Design review of the part built by this model. Coordinates are the model's own, in mm. A direction names the side the tool comes from. Coordinates: 2 decimals unless noted, no trailing zeros. Order: outer loops, then holes, each group sorted by start corner. A loop starts at its lowest first (then second) coordinate and runs counter-clockwise, first axis right, second up. Notation, with made-up numbers: M 82.25,27.5 L 115.25,27.5 A22 cw 115.25,41.5 Z; hole C 49.5,47 d6. An arc over 180 degrees is marked long. Answer as a JSON object with one key per item and string values.
from build123d import *

# Parameters (mm, degrees)
BOSS_EXTRUDE1_DEPTH = 50
CUT_EXTRUDE1_DEPTH  = 48
FILLET1_R           = 1
FILLET2_R           = 2
SKETCH3_R           = 1.6
CUT_EXTRUDE2_DEPTH  = 1067.768955656


with BuildPart() as part:
    # Sketch1 → Boss-Extrude1 (new body)
    with BuildSketch(Plane(origin=(0, 0, 0), x_dir=(1, 0, 0), z_dir=(0, 1, 0))):
        Polygon((1026.361248777, 29.83084978), (1061.002264928, 49.83084978), (1061.002264928, 99.83084978), (1049.002264928, 99.83084978), (1049.002264928, 56.75905301), (1026.361248777, 43.68725624), align=None)
    extrude(amount=BOSS_EXTRUDE1_DEPTH)

    # Sketch2 → Cut-Extrude1 (cut)
    with BuildSketch(Plane(origin=(0, 50, 0), x_dir=(1, 0, 0), z_dir=(0, 1, 0))):
        Polygon((1059.002264928, 99.83084978), (1059.002264928, 50.985550318), (1026.361248777, 32.140250857), (1013.240003321, 83.162287717), (1049.002264928, 102.282604927), align=None)
    extrude(amount=-CUT_EXTRUDE1_DEPTH, mode=Mode.SUBTRACT)

    # Fillet1
    fillet1_edges = [part.edges().sort_by_distance(p)[0] for p in [
        (1037.681756852, 2, -50.223154625),
        (1049.002264928, 2, -78.294951395),
        (1042.681756852, 50, -41.562900587),
        (1059.002264928, 50, -75.408200049),
    ]]
    fillet(fillet1_edges, radius=FILLET1_R)

    # Fillet2
    fillet2_edges = [part.edges().sort_by_distance(p)[0] for p in [
        (1059.002264928, 2, -75.408200049),
        (1042.681756852, 2, -41.562900587),
    ]]
    fillet(fillet2_edges, radius=FILLET2_R)

    # Sketch3 → Cut-Extrude2 (cut, through all)
    with BuildSketch(Plane(origin=(0, 2, 0), x_dir=(1, 0, 0), z_dir=(0, 1, 0))):
        with Locations(Location((1039.942264928, 46.332107148, 0), (0, 0, 270))):
            Circle(SKETCH3_R)
        with Locations(Location((1053.502264928, 59.83084978, 0), (0, 0, 270))):
            Circle(SKETCH3_R)
        with Locations(Location((1053.502264928, 89.83084978, 0), (0, 0, 270))):
            Circle(SKETCH3_R)
    extrude(amount=-CUT_EXTRUDE2_DEPTH, mode=Mode.SUBTRACT)


solid = part.part
1) Tool access review of faces 1 (the flat face through (1026.361, 19.3, -31.7)), 2 (the flat face through (1059.002, 27, -76)): name each direction out of +Z, -Z, +X, -X, +Y, -Y from which nothing blocks a thin tool from reaching the whole face with its end or side.
Taken from the geometry:
{"face 1": "+Z, -Z, -X, +Y, -Y", "face 2": "-Z, -X, +Y"}
2) To check wall thickness, follow L1, parallel to X at y = 8, z = -73.5; L2, parallel to Y at x = 1051.5, z = -91; L3, parallel to Z at x = 1050, y = 38. State the ranges of each line that lie inside material, in increasing order.
Taken from the geometry:
{"L1": "x = 1059 to 1061", "L2": "y = 0 to 2", "L3": "z = -45.79 to -43.48"}
3) Mouldability with a two-part tool opening along X and no side actions: class faces 3 (the cylindrical face through (1038.38, 1.01, -46.68)), 4 (the cylindrical face through (1058.4, 2.57, -75.07)), 5 (the flat face through (1043.44, 24.65, -39.69)) as released by +X, released by -X, zero draft, split by the parting line, or undercut.
Taken from the geometry:
{"face 3": "undercut", "face 4": "released by -X", "face 5": "released by +X"}
4) Add section B-B (z = -66). State the section outline as (x, y) points, and give its area (3 significant figures).
Taken from the geometry:
{"outline": "M 1049,0 L 1061,0 L 1061,50 L 1060,50 A1 ccw 1059,49 L 1059,4 A2 cw 1057,2 L 1050,2 A1 ccw 1049,1 Z", "area": "120 mm2"}
5) Add section A-A (y = 40). State the section outline as (x, z) points.
Taken from the geometry:
{"outline": "M 1026.36,-32.14 L 1059,-50.99 L 1059,-99.83 L 1061,-99.83 L 1061,-49.83 L 1026.36,-29.83 Z"}
6) Insertion check: pin 1 Ø8 at (y, z) = (36.5, -48.5) entering from +X; pin 2 Ø4 at (x, y) = (1048.5, 13) entering from -Z; pin 3 Ø10 at (x, z) = (1054, -38) entering from +Y; pin 4 Ø6 at (x, y) = (1052.5, 37) entering from +Z. Each pin has a flat end and moves straight along its axis. Give the tip position at first contact, or say it passes through.
Taken from the geometry:
{"pin 1": "stops at x = 1061", "pin 2": "stops at z = -46.08", "pin 3": "passes through", "pin 4": "stops at z = -43.19"}
